```python
from build123d import *

# Parameters (mm, degrees)
SKETCH1_W                         = 177.8
SKETCH1_H                         = 66.675
EXTRUDE1_DEPTH                    = 15.875
F_1_2_CLEARANCE_HOLE1_AT_2_COUNT  = 2
F_1_2_CLEARANCE_HOLE1_AT_2_PITCH  = 34.925
F_1_2_CLEARANCE_HOLE1_AT_3_COUNT  = 2
F_1_2_CLEARANCE_HOLE1_AT_3_PITCH  = 139.7
F_1_2_CLEARANCE_HOLE1_AT_4_COUNT  = 2
F_1_2_CLEARANCE_HOLE1_AT_4_PITCH  = 143.999463975
SKETCH15_W                        = 101.6
SKETCH15_H                        = 66.675
CUT_EXTRUDE1_DEPTH                = 1.016
CUT_EXTRUDE2_DEPTH                = 19.05
F_1_2_13_TAPPED_HOLE1_D           = 10.71626
F_1_2_13_TAPPED_HOLE1_DEPTH       = 14.859
F_1_2_13_TAPPED_HOLE1_CSINK_D     = 13.97
F_1_2_13_TAPPED_HOLE1_CSINK_ANGLE = 82


with BuildPart() as part:
    # Sketch1 → Extrude1 (new body)
    with BuildSketch(Plane.XY):
        with Locations((0, 33.3375)):
            Rectangle(SKETCH1_W, SKETCH1_H)
    extrude(amount=EXTRUDE1_DEPTH)

    # Sketch11 → 1/2 Clearance Hole1 (revolve, cut)
    with BuildSketch(Plane(origin=(-69.85, 50.8, 15.875), x_dir=(0, -1, 0), z_dir=(1, 0, 0))):
        Polygon((0, 0), (0, 15.875), (10.16, 15.875), (9.525, 15.144516061), (9.525, 0.730483939), (10.16, 0), align=None)
    f_1_2_clearance_hole1 = revolve(axis=Axis((-69.85, 50.8, 22.225), (0, 0, -1)), mode=Mode.SUBTRACT)

    # 1/2 Clearance Hole1 at 2: 1/2 Clearance Hole1 ×2
    with Locations(*[(0, -i * F_1_2_CLEARANCE_HOLE1_AT_2_PITCH, 0) for i in range(1, F_1_2_CLEARANCE_HOLE1_AT_2_COUNT)]):
        add(f_1_2_clearance_hole1, mode=Mode.SUBTRACT)

    # 1/2 Clearance Hole1 at 3: 1/2 Clearance Hole1 ×2
    with Locations(*[(i * F_1_2_CLEARANCE_HOLE1_AT_3_PITCH, 0, 0) for i in range(1, F_1_2_CLEARANCE_HOLE1_AT_3_COUNT)]):
        add(f_1_2_clearance_hole1, mode=Mode.SUBTRACT)

    # 1/2 Clearance Hole1 at 4: 1/2 Clearance Hole1 ×2
    with Locations(*[Vector(0.9701425, -0.242535625, 0) * (i * F_1_2_CLEARANCE_HOLE1_AT_4_PITCH) for i in range(1, F_1_2_CLEARANCE_HOLE1_AT_4_COUNT)]):
        add(f_1_2_clearance_hole1, mode=Mode.SUBTRACT)

    # Sketch15 → Cut-Extrude1 (cut)
    with BuildSketch(Plane(origin=(0, 0, 0), x_dir=(-1, 0, 0), z_dir=(0, 0, -1))):
        with Locations((0, 33.3375)):
            Rectangle(SKETCH15_W, SKETCH15_H)
    extrude(amount=-CUT_EXTRUDE1_DEPTH, mode=Mode.SUBTRACT)

    # Sketch17 → Cut-Extrude2 (cut, symmetric)
    with BuildSketch(Plane(origin=(0, 0, 0), x_dir=(0, 0, -1), z_dir=(1, 0, 0))):
        Polygon((-6.35, 0), (0, 10.998522628), (0, 0), align=None)
    extrude(amount=CUT_EXTRUDE2_DEPTH, both=True, mode=Mode.SUBTRACT)

    # 1/2-13 Tapped Hole1
    with Locations(Plane.XY.offset(15.875)):
        with Locations((0, 50.8), (0, 15.875)):
            CounterSinkHole(F_1_2_13_TAPPED_HOLE1_D / 2, F_1_2_13_TAPPED_HOLE1_CSINK_D / 2, depth=F_1_2_13_TAPPED_HOLE1_DEPTH, counter_sink_angle=F_1_2_13_TAPPED_HOLE1_CSINK_ANGLE)


solid = part.part
```
Here's how the part is built. I have some questions about the finished solid (model axes, mm). A direction names the side the tool comes from. Coordinates: 2 decimals unless noted, no trailing zeros. Order: outer loops, then holes, each group sorted by start corner. A loop starts at its lowest first (then second) coordinate and runs counter-clockwise, first axis right, second up. Notation, with made-up numbers: (27, 8) -> (43, 8) arc R21 ccw to (43, 15) -> close; hole circle Ø7 at (80.25, 79.5). An arc over 180 degrees is marked (long way). Return JSON: item names as keys, results as strings.
1) On a 3-axis mill with a long thin cutter (end or side, diameter ignored), from which of +Z, -Z, +X, -X, +Y, -Y can I reach the whole of each face in a straight line? I mean faces 1 (the flat face through (-19.05, 3, 2)), 2 (the flat face through (-70, 34, 0)), 3 (the flat face through (1, 34, 1.016)). Say none if no direction works.
Conclusion:
{"face 1": "-Z, -Y", "face 2": "-Z, +X, -X, +Y, -Y", "face 3": "-Z, +Y, -Y"}
2) If we section it at A-A on x = 0: State how many separate pieces and enclosed holes the cut face has, plus the area to 3 significant figures.
Conclusion:
{"separate pieces": "3", "enclosed holes": "0", "area": "642 mm²"}
3) If I drill on probe 1 along Y at (x, z) = (-69.85, 5) (3 decimals); probe 2 along Y at (x, z) = (0, 11.25) (3 decimals); probe 3 along X at (y, z) = (50.8, 10) (3 decimals), over which ranges is the centre line in solid material (lowest first)?
Conclusion:
{"probe 1": "y = 0 to 6.35, 25.4 to 41.275, 60.325 to 66.675", "probe 2": "y = 0 to 10.517, 21.233 to 45.442, 56.158 to 66.675", "probe 3": "x = -88.9 to -79.375, -60.325 to -5.358, 5.358 to 60.325, 79.375 to 88.9"}
4) I'm going to push a flat-ended pin straight in: P1, Ø3, axis at x = -45, y = 56.5, coming from the -Z side. Where does the tip first touch, or does it pass through?
Conclusion:
{"P1": "stops at z = 1.02"}
5) Thinking about a two-plate mould opening in Y: for faces 4 (the flat face through (-1, 66.675, 8)), 5 (the flat face through (-1, 34, 15.875)), 6 (the cylindrical face through (0.698, 56.113, 7.419)), which applies, +Y half, -Y half, draft (parallel to the pull), parting line (faces both ways), or undercut?
Conclusion:
{"face 4": "+Y half", "face 5": "draft", "face 6": "undercut"}
6) If we section it at D-D on x = -69.85: List the corners of the cut face in (y, z) for me (3 decimals).
Conclusion:
{"outline": "(0, 0) -> (5.715, 0) -> (6.35, 0.73) -> (6.35, 15.145) -> (5.715, 15.875) -> (0, 15.875) -> close; (25.4, 0.73) -> (26.035, 0) -> (40.64, 0) -> (41.275, 0.73) -> (41.275, 15.145) -> (40.64, 15.875) -> (26.035, 15.875) -> (25.4, 15.145) -> close; (60.325, 0.73) -> (60.96, 0) -> (66.675, 0) -> (66.675, 15.875) -> (60.96, 15.875) -> (60.325, 15.145) -> close"}
7) If we section it at C-C on z = 9: List the corners of the cut face in (x, y) for me (3 decimals), plus the area to 3 significant figures.
Conclusion:
{"outline": "(-88.9, 0) -> (88.9, 0) -> (88.9, 66.675) -> (-88.9, 66.675) -> close; hole circle Ø19.05 at (-69.85, 15.875); hole circle Ø19.05 at (-69.85, 50.8); hole circle Ø10.716 at (0, 15.875); hole circle Ø10.716 at (0, 50.8); hole circle Ø19.05 at (69.85, 15.875); hole circle Ø19.05 at (69.85, 50.8)", "area": "10,500 mm²"}
